For this review, take the finished solid that the model builds, in its own axes (mm). A direction names the side the tool comes from. Coordinates: 2 decimals unless noted, no trailing zeros. Loops run counter-clockwise (first coordinate to the right, second up) from the corner with the lowest first, then second, coordinate; pieces in that order, holes last. Notation, with made-up numbers: (40, 60.5) -> (96, 60.5) arc R10 ccw to (96, 69.5) -> close; hole circle Ø4 at (27.5, -11.75). An arc over 180 degrees is marked (long way). One line per item, written item: value.
from build123d import *

# Parameters (mm, degrees)
BOSS_EXTRUDE1_DEPTH = 34
SKETCH2_W           = 36
SKETCH2_H           = 30
CUT_EXTRUDE1_DEPTH  = 1.5
SKETCH3_W           = 36
SKETCH3_H           = 30
CUT_EXTRUDE2_DEPTH  = 1.5
SKETCH4_W           = 36
SKETCH4_H           = 30
CUT_EXTRUDE3_DEPTH  = 1.5
CUT_EXTRUDE5_DEPTH  = 31.5
SKETCH6_W           = 37.25
SKETCH6_H           = 1.921966438
BOSS_EXTRUDE2_DEPTH = 5
SKETCH7_W           = 37.25
SKETCH7_H           = 2.5
BOSS_EXTRUDE3_DEPTH = 5


with BuildPart() as part:
    # Sketch1 → Boss-Extrude1 (new body)
    with BuildSketch(Plane(origin=(0, 0, 0), x_dir=(1, 0, 0), z_dir=(0, 1, 0))):
        Polygon((20.323082913, -34.452464366), (39.998250821, 0.374073902), (19.675167908, 34.826538269), (-20.323082913, 34.452464366), (-39.998250821, -0.374073902), (-19.675167908, -34.826538269), align=None)
    extrude(amount=BOSS_EXTRUDE1_DEPTH)

    # Sketch2 → Cut-Extrude1 (cut)
    with BuildSketch(Plane(origin=(0.323957502, 0, 34.639501318), x_dir=(0.9999562705174567, 0, -0.00935184756179416), z_dir=(0.009351847561794161, 0, 0.9999562705174567))):
        with Locations((0.07819078, 17.042979031)):
            Rectangle(SKETCH2_W, SKETCH2_H)
    extrude(amount=-CUT_EXTRUDE1_DEPTH, mode=Mode.SUBTRACT)

    # Sketch3 → Cut-Extrude2 (cut)
    with BuildSketch(Plane(origin=(-0.323957502, 0, -34.639501318), x_dir=(-0.9999562705174567, 0, 0.009351847561793986), z_dir=(-0.009351847561793988, 0, -0.9999562705174567))):
        with Locations((-0.090906466, 17.061793862)):
            Rectangle(SKETCH3_W, SKETCH3_H)
    extrude(amount=-CUT_EXTRUDE2_DEPTH, mode=Mode.SUBTRACT)

    # Sketch4 → Cut-Extrude3 (cut)
    with BuildSketch(Plane(origin=(0, 34, 0), x_dir=(1, 0, 0), z_dir=(0, 1, 0))):
        Rectangle(SKETCH4_W, SKETCH4_H)
    extrude(amount=-CUT_EXTRUDE3_DEPTH, mode=Mode.SUBTRACT)

    # Sketch5 → Cut-Extrude5 (cut)
    with BuildSketch(Plane.XZ):
        Polygon((37.249997801, -0.012800837), (18.63608475, 32.253043968), (-18.61391305, 32.265844805), (-37.249997801, 0.012800837), (-18.63608475, -32.253043968), (18.61391305, -32.265844805), align=None)
    extrude(amount=-CUT_EXTRUDE5_DEPTH, mode=Mode.SUBTRACT)

    # Sketch6 → Boss-Extrude2 (add)
    with BuildSketch(Plane(origin=(27.943041275, 0, 16.120121566), x_dir=(-0.4997023637702259, 0, 0.8661971759607906), z_dir=(-0.8661971759607907, 0, -0.499702363770226))):
        with Locations((-0.009802695, 3.460983219)):
            Rectangle(SKETCH6_W, SKETCH6_H)
    extrude(amount=BOSS_EXTRUDE2_DEPTH)

    # Sketch7 → Boss-Extrude3 (add)
    with BuildSketch(Plane(origin=(-27.943041275, 0, -16.120121566), x_dir=(0.49970236377022564, 0, -0.8661971759607908), z_dir=(0.8661971759607908, 0, 0.49970236377022564))):
        with Locations((-0.003212365, 3.584418616)):
            Rectangle(SKETCH7_W, SKETCH7_H)
    extrude(amount=BOSS_EXTRUDE3_DEPTH)


solid = part.part
1. For faces 4 (the flat face through (0, 2.062, -34)), 5 (the flat face through (-28.073, 15.53, -15.894)), 6 (the flat face through (29.98, 16.76, -17.36)), 7 (the flat face through (27.8, 15.53, -16.37)), list the 3-axis set-ups (+Z, -Z, +X, -X, +Y, -Y) from which the entire face can be reached by the end or side of a thin tool; tool diameter is ignored.
Return value:
face 4: -Z
face 5: none
face 6: -Z, +X, +Y, -Y
face 7: -Y
2. Take a section at B-B, the plane z = 12. Give the boundary of the cut face in (x, y), and give its area (3 significant figures).
Return value:
outline: (-33.14, 0) -> (-30.32, 0) -> (-30.32, 31.5) -> (30.32, 31.5) -> (30.32, 4.42) -> (24.55, 4.42) -> (24.55, 2.5) -> (30.32, 2.5) -> (30.32, 0) -> (33.01, 0) -> (33.01, 34) -> (18, 34) -> (18, 32.5) -> (-18, 32.5) -> (-18, 34) -> (-33.14, 34) -> close
area: 296 mm2
3. Take a section at A-A, the plane y = 30. Give the boundary of the cut face in (x, z).
Return value:
outline: (-40, 0.37) -> (-20.32, -34.45) -> (-18.23, -34.47) -> (-18.22, -32.97) -> (17.78, -33.31) -> (17.77, -34.81) -> (19.68, -34.83) -> (40, -0.37) -> (20.32, 34.45) -> (18.4, 34.47) -> (18.39, 32.97) -> (-17.61, 33.31) -> (-17.6, 34.81) -> (-19.68, 34.83) -> close; hole (-37.25, 0.01) -> (-18.64, -32.25) -> (18.61, -32.27) -> (37.25, -0.01) -> (18.64, 32.25) -> (-18.61, 32.27) -> close
4. Take a section at D-D, the plane z = 27.5. Give the boundary of the cut face in (x, y), and give its area (3 significant figures).
Return value:
outline: (-24, 0) -> (-21.37, 0) -> (-21.37, 31.5) -> (21.38, 31.5) -> (21.38, 4.42) -> (15.61, 4.42) -> (15.61, 2.5) -> (21.38, 2.5) -> (21.38, 0) -> (24.25, 0) -> (24.25, 34) -> (-24, 34) -> close
area: 305 mm2
5. To check wall thickness, follow probe 1 along Y at (x, z) = (28, -1); probe 2 along Y at (x, z) = (7.5, 9.5); probe 3 along Z at (x, y) = (-8, 10.5). State the ranges of each line that lie inside material, in increasing order. Write a range as from..to.
Return value:
probe 1: y = 31.5..34
probe 2: y = 31.5..32.5
probe 3: z = -33.07..-32.26, 32.26..33.22
6. Take a section at C-C, the plane x = 0.5. Give the boundary of the cut face in (y, z).
Return value:
outline: (0, -34.65) -> (2.06, -34.65) -> (2.06, -33.15) -> (32.06, -33.15) -> (32.06, -34.65) -> (34, -34.65) -> (34, -15) -> (32.5, -15) -> (32.5, 15) -> (34, 15) -> (34, 34.64) -> (32.04, 34.64) -> (32.04, 33.14) -> (2.04, 33.14) -> (2.04, 34.64) -> (0, 34.64) -> (0, 32.26) -> (31.5, 32.26) -> (31.5, -32.26) -> (0, -32.26) -> close
7. The part is to be moulded in two halves that separate along X. For faces 1 (the flat face through (29, 0, 15)), 2 (the flat face through (0, 32.043, 34)), 3 (the flat face through (-30.023, 16.762, -17.283)), say which applies: pulls with the +X half, pulls with the -X half, needs draft (parallel to the pull), parting line crosses it, or undercut.
Return value:
face 1: needs draft
face 2: undercut
face 3: pulls with the -X half
8. Insertion check: pin 1 Ø5 at (x, y) = (21, 11) entering from +Z; pin 2 Ø5 at (y, z) = (15.5, 4.5) entering from +X; pin 3 Ø1.5 at (y, z) = (20.5, -25.5) entering from -X. Each pin has a flat end and moves straight along its axis. Give the tip position at first contact, or say it passes through.
Return value:
pin 1: stops at z = 34.47
pin 2: stops at x = 38.66
pin 3: stops at x = -25.8
